Autodesk Inventor part; units mm, degrees
ref_plane "YZ Plane" through (0, 0, 0) normal (1, 0, 0) x (0, 1, 0)
ref_plane "XZ Plane" through (0, 0, 0) normal (0, 1, 0) x (-1, 0, 0)
ref_plane "XY Plane" through (0, 0, 0) normal (0, 0, 1) x (1, 0, 0)
sketch "Skizze1" plane through (0, 0, 0) normal (0, 0, 1) x (1, 0, 0)
  circle A0 centre (0, 0) radius 30
  dimension "d0" = 60
extrude "Extrusion1" add sketch "Skizze1" along normal blind 10
sketch "Skizze2" plane through (0, 0, 10) normal (0, 0, 1) x (1, 0, 0)
  circle A0 centre (0, 0) radius 30
  circle A1 centre (0, 0) radius 22.5
  circle A2 centre (0, 0) radius 5
  dimension "d3" = 7.5
  dimension "d4" = 10
extrude "Extrusion2" cut sketch "Skizze2" against normal blind 7 contours A1
sketch "Skizze3" plane through (0, 0, 10) normal (0, 0, 1) x (1, 0, 0)
  circle A0 centre (0, 0) radius 1
  dimension "d7" = 2
extrude "Extrusion3" cut sketch "Skizze3" along normal through all both and the other way through all
fillet "Rundung1" radius 0.2 2 edges at (-22.5, 0, 3) (-5, 0, 3)
chamfer "Fase1" distance 0.2 angle 45 6 edges at (-30, 0, 0) (-30, 0, 10) (-22.5, 0, 10) (-5, 0, 10) (-1, 0, 10) (-1, 0, 0)
sketch "Skizze4" plane through (0, 0, 10) normal (0, 0, 1) x (1, 0, 0)
  circle A0 centre (0, 0) radius 25
  circle A1 centre (0, 0) radius 40
  dimension "d14" = 50
  dimension "d15" = 15
extrude "Extrusion4" cut sketch "Skizze4" along normal through all both and the other way through all
sketch "Skizze5" plane through (0, 0, 10) normal (0, 0, 1) x (1, 0, 0)
  circle A0 centre (0, 0) radius 1.2
  circle A1 centre (0, 0) radius 27.5
  circle A2 centre (0, 0) radius 30
  dimension "d18" = 55
  dimension "d19" = 60
properties part number "felge" material "Aluminium 6061"
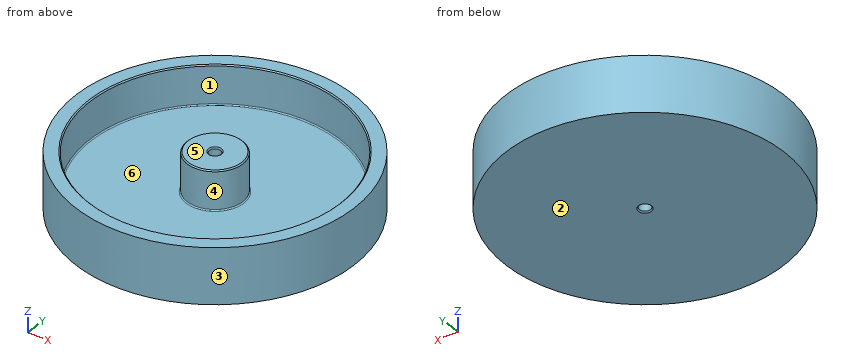
Geometry: final body of the model. Coordinates: model frame, mm. Face numbers are marked on the shaded views. A direction names the side the tool comes from. Give positions to 0.01 mm unless a question says otherwise; leave off trailing zeros. Write each loop counter-clockwise with the first axis right and the second up, starting at its lowest first coordinate (ties: lowest second). Pieces come first, ordered by that corner, then holes.
1. Draft query along Y for the marked faces 1, 2, 3 and 4. Return one class per face: released by +Y, released by -Y, zero draft, split by the parting line, or undercut.
2. Section query A-A, the plane y = 0. Return loops of the section in (x, z), then the cut area to 3 significant figures.
3. Section query D-D, the plane z = 2.25. Return loops of the section in (x, y).
4. Pin query (flat end, axial travel): P1, Ø6, axis at y = -4.5, z = 8.5, coming from the -X side; P2, Ø5, axis at x = -10.5, z = 4, coming from the +Y side; P3, Ø2, axis at y = -20, z = 8.5, coming from the +X side. Return the tip coordinate at first contact, or that it passes through.
5. Line query: probe 1 along Y at (x, z) = (0, 8.25); probe 2 along Y at (x, z) = (-4, 5); probe 3 along Z at (x, y) = (-6, 11.5). Output: solid intervals per line, ascending.
6. Reachability of the marked faces 5 and 6 from +Z, -Z, +X, -X, +Y, -Y: full face, straight path, thin tool, end or side. Return the list, or none.
7. Section query C-C, the plane z = 7.5. Return loops of the section in (x, y).
Computed:
1. face 1: undercut
1. face 2: zero draft
1. face 3: split by the parting line
1. face 4: undercut
2. outline: (-25, 0) - (-1.2, 0) - (-1, 0.2) - (-1, 9.8) - (-1.2, 10) - (-4.8, 10) - (-5, 9.8) - (-5, 3.2) arc R0.2 cw to (-5.2, 3) - (-22.3, 3) arc R0.2 cw to (-22.5, 3.2) - (-22.5, 9.8) - (-22.7, 10) - (-25, 10) - close; (1, 0.2) - (1.2, 0) - (25, 0) - (25, 10) - (22.7, 10) - (22.5, 9.8) - (22.5, 3.2) arc R0.2 cw to (22.3, 3) - (5.2, 3) arc R0.2 cw to (5, 3.2) - (5, 9.8) - (4.8, 10) - (1.2, 10) - (1, 9.8) - close
2. area: 235 mm2
3. outline: circle Ø50 at (0, 0); hole circle Ø2 at (0, 0)
4. P1: stops at x = -24.95
4. P2: stops at y = 23.69
4. P3: stops at x = 16.25
5. probe 1: y = -25 to -22.5, -5 to -1, 1 to 5, 22.5 to 25
5. probe 2: y = -24.68 to -22.14, -3 to 3, 22.14 to 24.68
5. probe 3: z = 0 to 3
6. face 5: +Z, +X, -X, +Y, -Y
6. face 6: +Z
7. outline: circle Ø50 at (0, 0); circle Ø10 at (0, 0); hole circle Ø45 at (0, 0); hole circle Ø2 at (0, 0)
